Check sheet for the modelled part. Datum: model origin and axes. Units: mm. A direction names the side the tool comes from. Coordinates: 2 decimals unless noted, no trailing zeros. Order: outer loops, then holes, each group sorted by start corner. A loop starts at its lowest first (then second) coordinate and runs counter-clockwise, first axis right, second up.
Autodesk Inventor part; units mm, degrees
ref_plane "YZ Plane" through (0, 0, 0) normal (1, 0, 0) x (0, 1, 0)
ref_plane "XZ Plane" through (0, 0, 0) normal (0, 1, 0) x (-1, 0, 0)
ref_plane "XY Plane" through (0, 0, 0) normal (0, 0, 1) x (1, 0, 0)
sketch "Sketch1" plane through (0, 0, 0) normal (0, 1, 0) x (-1, 0, 0)
  circle A0 centre (0, 0) radius 25
  line L0 (0, 0) -> (20, 0)
  circle A1 centre (20, 0) radius 5
  line L1 (7.5, 45) -> (-7.5, 45)
  line L2 (-7.5, 45) -> (-7.5, -45)
  line L3 (-7.5, -45) -> (7.5, -45)
  line L4 (7.5, -45) -> (7.5, 45)
  line L5 (7.5, 45) -> (-7.5, -45) construction
  line L6 (-7.5, 45) -> (7.5, -45) construction
  point P0 (7.5, 23.8485)
  point P1 (-7.5, 23.8485)
  point P2 (-7.5, -23.8485)
  point P3 (7.5, -23.8485)
  dimension "d0" = 50
  dimension "d1" = 20
  dimension "d2" = 10
  dimension "d3" = 15
  dimension "d4" = 90
extrude "Extrusion1" add sketch "Sketch1" along normal blind 10 contours A1 L0 L4 A0 | A1 | A0 L4 L0 A1 | L4 A0 L2 | L2 A0
extrude "Extrusion2" cut sketch "Sketch1" along normal blind 25 contours A1
extrude "Extrusion3" cut sketch "Sketch1" along normal blind 3 contours L4 A0 L2
sketch "Sketch2" plane through (0, 10, 0) normal (0, 1, 0) x (1, 0, 0)
  circle A0 centre (0, 0) radius 5
  circle A1 centre (0, 0) radius 2.25
  dimension "d11" = 10
  dimension "d12" = 4.5
extrude "Extrusion4" add sketch "Sketch2" along normal blind 25
fillet "Fillet1" radius 5 1 edges at (-5, 10, 0)
properties part number "GUIA GIRATORIA"
(1) Thickness scan on probe 1 along X at (y, z) = (18.25, 0); probe 2 along Y at (x, z) = (-12, 4.5). Record the ranges inside material, lowest first.
Filled in:
probe 1: x = -5 to -2.25, 2.25 to 5
probe 2: y = 0 to 10
(2) Cross-section at D-D (z = -16.5). Enter the section's corners in (x, y), and give its area (3 significant figures).
Filled in:
outline: (-18.78, 0) - (-7.5, 0) - (-7.5, 3) - (7.5, 3) - (7.5, 0) - (18.78, 0) - (18.78, 10) - (-18.78, 10) - close
area: 331 mm2
(3) Go/stop test with flat-tipped pins: P1, Ø1.5, axis at y = 2, z = 3, coming from the +X side; P2, Ø10, axis at x = 1, z = -14, coming from the +Y side; P3, Ø7.5, axis at x = 3.5, z = -5, coming from the -Y side; P4, Ø10, axis at x = -14.5, y = 17.5, coming from the +Z side. Record where each tip stops, or that it passes through.
Filled in:
P1: stops at x = 24.9
P2: stops at y = 10.09
P3: stops at y = 3
P4: passes through
(4) Release check for a two-part mould opening along Z. For faces 1 (the flat face through (0, 10, 0)), 2 (the flat face through (0, 10, -11)), 3 (the cylindrical face through (-1.08, 24.86, -4.88)) record: +Z half, -Z half, draft (parallel to the pull), parting line (faces both ways), or undercut.
Filled in:
face 1: undercut
face 2: draft
face 3: parting line
(5) Cross-section at A-A (x = -20). Enter the section's corners in (y, z).
Filled in:
outline: (0, -15) - (10, -15) - (10, -5) - (0, -5) - close; (0, 5) - (10, 5) - (10, 15) - (0, 15) - close
(6) Cross-section at C-C (y = 21.5). Enter the section's corners in (x, z).
Filled in:
outline: circle Ø10 at (0, 0); hole circle Ø4.5 at (0, 0)
(7) Tool access check on faces 4 (the flat face through (7.5, 1, 0)), 5 (the cylindrical face through (-0.29, 22.32, 2.23)), 6 (the flat face through (14, 0, 0)). Record the directions out of +Z, -Z, +X, -X, +Y, -Y that give a thin tool (end or side, any length) a straight path to the whole face; none if there is none.
Filled in:
face 4: +Z, -Z, -Y
face 5: +Y
face 6: +Z, -Z, +X, -X, -Y
(8) Cross-section at B-B (x = 0). Enter the section's corners in (y, z).
Filled in:
outline: (3, -25) - (10, -25) - (10, -10) arc R5 cw to (15, -5) - (35, -5) - (35, -2.25) - (10, -2.25) - (10, 2.25) - (35, 2.25) - (35, 5) - (15, 5) arc R5 cw to (10, 10) - (10, 25) - (3, 25) - close
